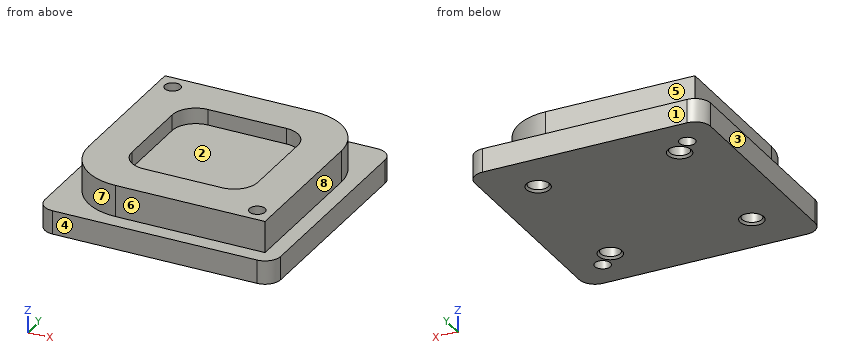
Autodesk Inventor part; units mm, degrees
ref_plane "YZ Plane" through (0, 0, 0) normal (1, 0, 0) x (0, 1, 0)
ref_plane "XZ Plane" through (0, 0, 0) normal (0, 1, 0) x (-1, 0, 0)
ref_plane "XY Plane" through (0, 0, 0) normal (0, 0, 1) x (1, 0, 0)
sketch "Sketch1" plane through (0, 0, 0) normal (0, 0, 1) x (1, 0, 0)
  line L0 (-47.625, 47.625) -> (47.625, 47.625)
  line L1 (47.625, 47.625) -> (47.625, -47.625)
  line L2 (47.625, -47.625) -> (-47.625, -47.625)
  line L3 (-47.625, -47.625) -> (-47.625, 47.625)
  line L4 (-47.625, 47.625) -> (47.625, -47.625) construction
  line L5 (47.625, 47.625) -> (-47.625, -47.625) construction
  point P0 (0, 0)
  dimension "d0" = 95.25
  dimension "d1" = 95.25
extrude "Extrusion1" add sketch "Sketch1" along normal blind 9.525
sketch "Sketch2" plane through (0, 0, 9.525) normal (0, 0, 1) x (1, 0, 0)
  line L0 (41.275, -41.275) -> (-41.275, -41.275)
  line L1 (-41.275, -41.275) -> (-41.275, 41.275)
  line L2 (-41.275, 41.275) -> (41.275, 41.275)
  line L3 (41.275, 41.275) -> (41.275, -41.275)
  line L4 (41.275, -41.275) -> (-41.275, 41.275) construction
  line L5 (-41.275, -41.275) -> (41.275, 41.275) construction
  point P0 (0, 0)
  dimension "d4" = 82.55
  dimension "d5" = 82.55
extrude "Extrusion2" add sketch "Sketch2" along normal blind 12.7
sketch "Sketch3" plane through (0, 0, 22.225) normal (0, 0, 1) x (1, 0, 0)
  line L0 (-25.4, -25.4) -> (25.4, -25.4)
  line L1 (25.4, -25.4) -> (25.4, 25.4)
  line L2 (25.4, 25.4) -> (-25.4, 25.4)
  line L3 (-25.4, 25.4) -> (-25.4, -25.4)
  line L4 (-25.4, -25.4) -> (25.4, 25.4) construction
  line L5 (25.4, -25.4) -> (-25.4, 25.4) construction
  point P0 (0, 0)
  dimension "d8" = 50.8
  dimension "d9" = 50.8
extrude "Extrusion3" cut sketch "Sketch3" against normal blind 6.35
sketch "Sketch4" plane through (0, 0, 22.225) normal (0, 0, 1) x (1, 0, 0)
  line L0 (-41.275, 41.275) -> (-41.275, -41.275)
  line L1 (41.275, 41.275) -> (-41.275, 41.275)
  line L2 (-41.275, -41.275) -> (41.275, -41.275)
  line L3 (41.275, -41.275) -> (41.275, 41.275)
  point P0 (0, 0)
  point P1 (-34.925, 34.925)
  point P2 (34.925, -34.925)
  dimension "d19" = 6.35
  dimension "d20" = 6.35
  dimension "d21" = 6.35
  dimension "d22" = 6.35
hole "Hole1" at (-34.925, 34.925, 22.225) at (34.925, -34.925, 22.225) direction (0, 0, -1) diameter 6.35 end through all
sketch "Sketch5" plane through (0, 0, 0) normal (0, 0, -1) x (-1, 0, 0)
  point P0 (0, 0)
  point P1 (-28.575, 28.575)
  point P2 (28.575, 28.575)
  point P3 (28.575, -28.575)
  point P4 (-28.575, -28.575)
  dimension "d37" = 57.15
  dimension "d38" = 28.575
  dimension "d39" = 57.15
  dimension "d40" = 28.575
  dimension "d41" = 57.15
  dimension "d42" = 57.15
  dimension "d43" = 28.575
  dimension "d44" = 28.575
hole "Hole2" at (28.575, 28.575, 0) at (-28.575, 28.575, 0) at (-28.575, -28.575, 0) at (28.575, -28.575, 0) direction (0, 0, 1) diameter 7.9502 depth 15.875 tip angle 118 countersink diameter 9.525 countersink angle 82
fillet "Fillet1" radius 6.35 4 edges at (47.625, -47.625, 4.7625) (-47.625, -47.625, 4.7625) (47.625, 47.625, 4.7625) (-47.625, 47.625, 4.7625)
fillet "Fillet3" radius 22.225 2 edges at (41.275, 41.275, 15.875) (-41.275, -41.275, 15.875)
fillet "Fillet4" radius 9.525 4 edges at (-25.4, 25.4, 19.05) (-25.4, -25.4, 19.05) (25.4, 25.4, 19.05) (25.4, -25.4, 19.05)
thread "Thread1"
thread "Thread2"
thread "Thread3"
thread "Thread4"
properties part number "KUMAR_ACT6_L1" material "Aluminum 6061"
Input: part model. Units: mm. Frame: model coordinates. Face numbers are marked on the shaded views. A direction names the side the tool comes from. Give positions to 0.01 mm unless a question says otherwise; leave off trailing zeros. Order: outer loops, then holes, each group sorted by start corner. A loop starts at its lowest first (then second) coordinate and runs counter-clockwise, first axis right, second up. Notation, with made-up numbers: (39.5, 61.5) - (78.5, 61.5) arc R22 cw to (78.5, 70.5) - close; hole circle Ø7 at (11, 23). An arc over 180 degrees is marked (long way). One line per item, written item: value.
1. Reachability of the marked faces 5, 6, 7 and 8 from +Z, -Z, +X, -X, +Y, -Y: full face, straight path, thin tool, end or side. Return the list, or none.
Determined:
face 5: +Z, +X, -X, +Y
face 6: +Z, +X, -X, -Y
face 7: +Z, -X, -Y
face 8: +Z, +X, +Y, -Y
2. Cut plane C-C, the plane y = 5. Output: boundary loops of the cut face in (x, z) (3 decimals).
Determined:
outline: (-47.625, 0) - (47.625, 0) - (47.625, 9.525) - (41.275, 9.525) - (41.275, 22.225) - (25.4, 22.225) - (25.4, 15.875) - (-25.4, 15.875) - (-25.4, 22.225) - (-41.275, 22.225) - (-41.275, 9.525) - (-47.625, 9.525) - close
3. Draft query along Y for the marked faces 1, 2, 3 and 4. Return one class per face: released by +Y, released by -Y, zero draft, split by the parting line, or undercut.
Determined:
face 1: released by +Y
face 2: undercut
face 3: zero draft
face 4: released by -Y
4. Line query: probe 1 along X at (y, z) = (13, 20.25) (3 decimals); probe 2 along Z at (x, y) = (-12, -42.5) (3 decimals); probe 3 along Z at (x, y) = (-16.5, -12) (3 decimals). Output: solid intervals per line, ascending.
Determined:
probe 1: -41.275 to -25.4, 25.4 to 41.275
probe 2: 0 to 9.525
probe 3: 0 to 15.875
5. Cut plane A-A, the plane x = 37. Output: boundary loops of the cut face in (y, z) (3 decimals), and give its area (3 significant figures).
Determined:
outline: (-47.625, 0) - (-37.328, 0) - (-37.328, 22.225) - (-41.275, 22.225) - (-41.275, 9.525) - (-47.625, 9.525) - close; (-32.522, 0) - (47.625, 0) - (47.625, 9.525) - (32.155, 9.525) - (32.155, 22.225) - (-32.522, 22.225) - close
area: 1,730 mm2
6. Cut plane B-B, the plane z = 6.5. Output: boundary loops of the cut face in (x, y) (3 decimals).
Determined:
outline: (-47.625, -41.275) arc R6.35 ccw to (-41.275, -47.625) - (41.275, -47.625) arc R6.35 ccw to (47.625, -41.275) - (47.625, 41.275) arc R6.35 ccw to (41.275, 47.625) - (-41.275, 47.625) arc R6.35 ccw to (-47.625, 41.275) - close; hole circle Ø6.35 at (-34.925, 34.925); hole circle Ø7.95 at (-28.575, -28.575); hole circle Ø7.95 at (-28.575, 28.575); hole circle Ø7.95 at (28.575, -28.575); hole circle Ø7.95 at (28.575, 28.575); hole circle Ø6.35 at (34.925, -34.925)
7. Pin query (flat end, axial travel): pin 1 Ø1.5 at (y, z) = (8, 19.5) entering from -X (3 decimals); pin 2 Ø5 at (x, z) = (-0.5, 19.5) entering from +Y (3 decimals); pin 3 Ø6 at (y, z) = (29.5, 18.5) entering from +X. Return the tip coordinate at first contact, or that it passes through.
Determined:
pin 1: x = -41.275
pin 2: y = 41.275
pin 3: x = 39.99
